```python
from build123d import *

# Parameters (mm, degrees)
F3_DEPTH = 8
F4_DEPTH = 8
F5_COUNT = 22


with BuildPart() as f3:
    # F2 (on offset) → F3 (new body)
    with BuildSketch(Plane.XY.offset(-9)):
        with BuildLine():
            ThreePointArc((14.5934619862, 3.4685540585), (-14.8980188245, -1.7461486487), (15, 0))
            ThreePointArc((15, 0), (14.8980188245, 1.7461486487), (14.5934619862, 3.4685540585))
        make_face()
        Polygon((-2.4537386441, -4.1687808289), (-4.9074772881, 0.0812191711), (-2.4537386441, 4.3312191711), (2.4537386441, 4.3312191711), (4.9074772881, 0.0812191711), (2.4537386441, -4.1687808289), align=None, mode=Mode.SUBTRACT)
        Polygon((-2.4537386441, 4.3312191711), (-4.9074772881, 0.0812191711), (-2.4537386441, -4.1687808289), (2.4537386441, -4.1687808289), (4.9074772881, 0.0812191711), (2.4537386441, 4.3312191711), align=None)
    extrude(amount=-F3_DEPTH)

    # F2 (on offset) → F4 (join, through all)
    with BuildSketch(Plane.XY.offset(-9)):
        with BuildLine():
            ThreePointArc((14.5934619862, 3.4685540585), (14.8980188245, 1.7461486487), (15, 0))
            ThreePointArc((15, 0), (15.6209528999, 1.8308814158), (14.5934619862, 3.4685540585))
        make_face()
    extrude(amount=-F4_DEPTH)

    # F5: F3 ×22 about axis
    f5_axis = Axis((0, 0, -9), (0, 0, 1))


with BuildPart() as f3_1:
    add(f3.part)
    for i in range(1, F5_COUNT):
        add(f3.part.rotate(f5_axis, i * 360 / F5_COUNT))

    # F0 (on Top) → F6 section 0
    with BuildSketch(Plane.XY):
        Polygon((-4.6188021535, 0), (-2.3094010768, -4), (2.3094010768, -4), (4.6188021535, 0), (2.3094010768, 4), (-2.3094010768, 4), align=None)
    # F2 (on offset) → F6 section 1
    with BuildSketch(Plane.XY.offset(-9)):
        Polygon((-2.4537386441, 4.3312191711), (-4.9074772881, 0.0812191711), (-2.4537386441, -4.1687808289), (2.4537386441, -4.1687808289), (4.9074772881, 0.0812191711), (2.4537386441, 4.3312191711), align=None)
    loft()


solid = f3_1.part
```
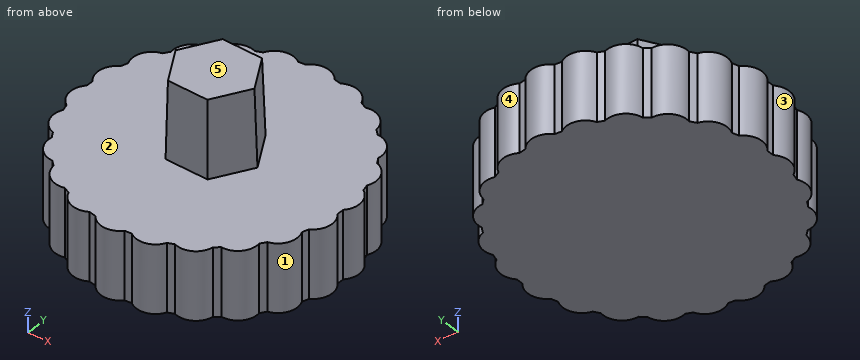
Read the model definition and answer for the solid it produces. Units are mm, in the model's axes. Face numbers are marked on the shaded views. A direction names the side the tool comes from. Coordinates: 2 decimals unless noted, no trailing zeros. Loops run counter-clockwise (first coordinate to the right, second up) from the corner with the lowest first, then second, coordinate; pieces in that order, holes last.
(1) A tool of negligible diameter and unlimited length cuts with its end or side. For the marked faces 1 and 2, from which of +Z, -Z, +X, -X, +Y, -Y can it reach the whole face along a straight path? Write none if from no direction.
Solution:
face 1: +Z, -Z, +X
face 2: +Z
(2) Flat-ended cylindrical pins translate along their axes: pin 1 Ø6 at (x, z) = (2.5, -7) entering from -Y; pin 2 Ø5 at (y, z) = (-8.5, -11.5) entering from +X; pin 3 Ø10 at (x, z) = (7, -10) entering from +Y; pin 4 Ø10 at (x, y) = (-1.5, -2.5) entering from +Z. Find the tip coordinate at first contact, or state that the pin passes through.
Solution:
pin 1: stops at y = -15.64
pin 2: stops at x = 14.36
pin 3: stops at y = 15.08
pin 4: stops at z = 0
(3) The mould has two halves that part along X. Classify the marked faces 3, 4 and 5: released by +X, released by -X, zero draft, split by the parting line, or undercut.
Solution:
face 3: released by -X
face 4: undercut
face 5: zero draft
(4) Consider line 1 along X through (y, z) = (9, -10.75); line 2 along Z through (x, y) = (-5, 9.5); line 3 along X through (y, z) = (5.5, -15.5). Determine where each line is inside the solid, lowest interval first.
Solution:
line 1: x = -12.2 to 12.62
line 2: z = -17 to -9
line 3: x = -14.32 to 14.64
(5) The part is cut by section A-A (y = 7). Determine the outline of the cut face in (x, z).
Solution:
outline: (-14.08, -17) - (13.85, -17) - (13.85, -9) - (-14.08, -9) - close
